Answer from the drawing. Dimensions are ordinates in mm from the lowest x, y and z of the part. A direction names the side the tool comes from. Give positions to 0.01 mm unless a question says otherwise; leave off trailing zeros. Order: outer loops, then holes, each group sorted by start corner. A loop starts at its lowest first (then second) coordinate and runs counter-clockwise, first axis right, second up. Notation, with made-up numbers: (46, 65.25) -> (95, 65.25) arc R25 ccw to (95, 82.25) -> close; hole circle Ø3 at (0, 16.5). An arc over 180 degrees is marked (long way). Write item = value, one per line. Start each with the question number.
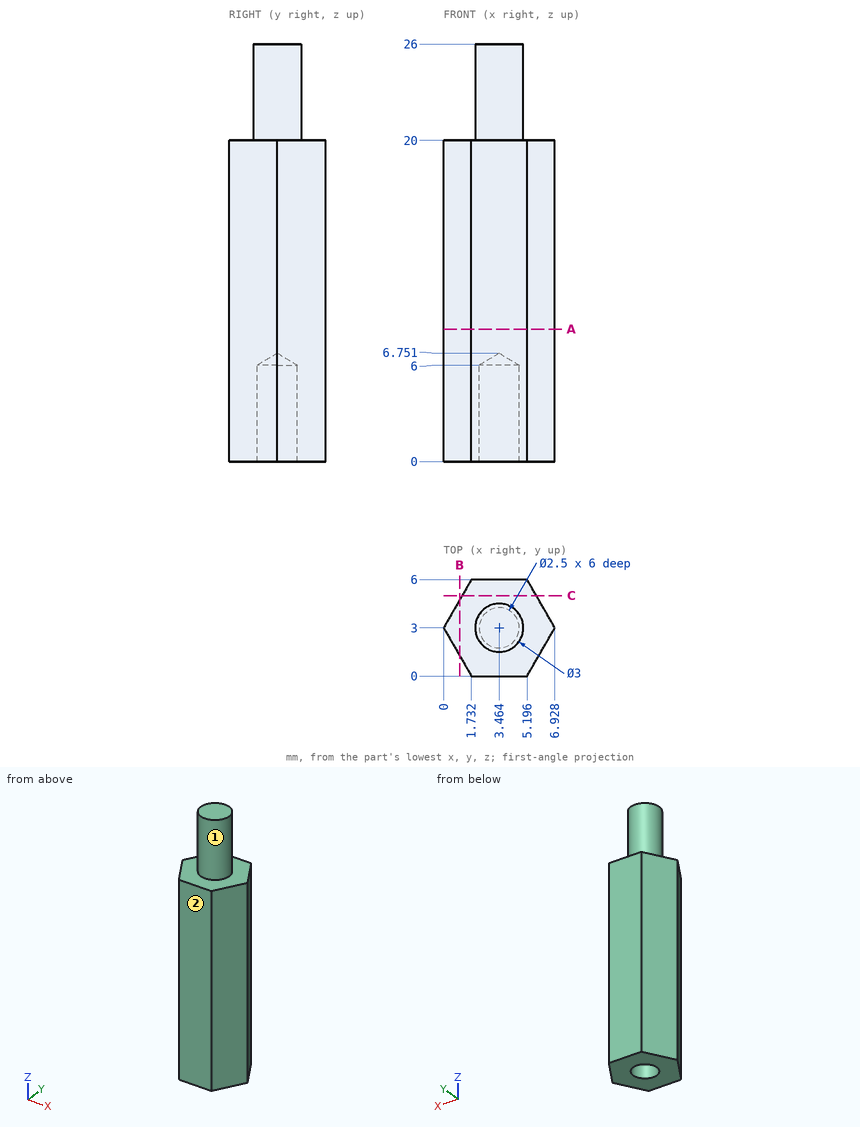
Item 1: A cutting plane is placed at B-B, the plane x = 1. Write down the section's boundary in (y, z).
Item 2: Flat-ended cylindrical pins translate along their axes: pin 1 (1.5 mm diameter, centred on y = 2, z = 4, fed in from +X); pin 2 (3 mm diameter, centred on x = 3.46, y = 3, fed in from -Z). Find the tip coordinate at first contact, or state that the pin passes through.
Item 3: Consider L1, parallel to Z at x = 4.5, y = 4.25; L2, parallel to X at y = 5.5, z = 16.5 (1 decimal); L3, parallel to Y at x = 4.25, z = 22.25. Determine where each line is inside the solid, lowest interval first. Write a range as from..to.
Item 4: A cutting plane is placed at C-C, the plane y = 5. Write down the section's boundary in (x, z) (1 decimal).
Item 5: A cutting plane is placed at A-A, the plane z = 8.25. Write down the section's boundary in (x, y), plus the area to 3 significant figures.
Item 6: Which of the six approach directions +Z, -Z, +X, -X, +Y, -Y give full straight-line access (tool end or side, diameter ignored) to the marked faces 1 and 2?
Check values:
q1.outline = (1.27, 0) -> (4.73, 0) -> (4.73, 20) -> (1.27, 20) -> close
q2.pin_1 = 6.78
q2.pin_2 = 0
q3.L1 = 0..20
q3.L2 = 1.4..5.5
q3.L3 = 1.72..4.28
q4.outline = (1.2, 0) -> (5.8, 0) -> (5.8, 20) -> (1.2, 20) -> close
q5.outline = (0, 3) -> (1.73, 0) -> (5.2, 0) -> (6.93, 3) -> (5.2, 6) -> (1.73, 6) -> close
q5.area = 31.2 mm^2
q6.face_1 = +Z
q6.face_2 = +Z, -Z, +X, -X, -Y
